Verification items for the finished model (mm, model axes). Face numbers are marked on the shaded views. Coordinates: 2 decimals unless noted, no trailing zeros. Write each loop counter-clockwise with the first axis right and the second up, starting at its lowest first coordinate (ties: lowest second). Pieces come first, ordered by that corner, then holes. Notation, with made-up numbers: (68.25, 71) -> (73.25, 71) arc R13 ccw to (73.25, 93) -> close; hole circle Ø10 at (71, -29). An arc over 180 degrees is marked (long way). Write item = value, one per line. Start each with the question number.
(1) Gauge pin test, flat ends, axial feed: pin 1 Ø3 at (y, z) = (-17, 3.5) entering from -X; pin 2 Ø2 at (y, z) = (33.5, 6) entering from -X. Record the tip position at first contact, or that the pin passes through.
(2) Mould release check, pull along X, two halves, no side actions. Record for the marked faces 1, 2 and 3: released by +X, released by -X, zero draft, split by the parting line, or undercut.
(3) Section check A-A (y = 0). State how many separate pieces and enclosed holes the cut face has, plus the area to 3 significant figures.
(4) Material ranges on probe 1 along Y at (x, z) = (25, 8); probe 2 along X at (y, z) = (7.5, 8); probe 3 along X at (y, z) = (-20, 6), recorded low to high. Write a range as [from, to].
(5) Section check B-B (z = 3.75). Record the cut outline in (x, y).
Autodesk Inventor part; units mm, degrees
ref_plane "YZ Plane" through (0, 0, 0) normal (1, 0, 0) x (0, 1, 0)
ref_plane "XZ Plane" through (0, 0, 0) normal (0, 1, 0) x (-1, 0, 0)
ref_plane "XY Plane" through (0, 0, 0) normal (0, 0, 1) x (1, 0, 0)
sketch "Sketch1" plane through (0, 0, 0) normal (0, 0, 1) x (1, 0, 0)
  circle A0 centre (0, 0) radius 46
  circle A1 centre (0, 0) radius 29.05
  dimension "d0" = 58.1
  dimension "d1" = 92
extrude "Extrusion1" add sketch "Sketch1" along normal blind 10
sketch "Sketch2" plane through (0, 0, 10) normal (0, 0, 1) x (1, 0, 0)
  circle A0 centre (0, 0) radius 29.05
  circle A1 centre (0, 0) radius 40 construction
  point P0 (0, 40)
  dimension "d4" = 80
hole "Hole1" at (0, 40, 10) direction (0, 0, -1) diameter 6.5 end through all
pattern_circular "Circular Pattern1" count 4 over 360 about axis through (0, 0, 0) along (0, 0, 1) of "Hole1"
sketch "Sketch4" plane through (0, 0, 10) normal (0, 0, 1) x (1, 0, 0)
  circle A0 centre (0, 0) radius 30
  circle A1 centre (0, 0) radius 34
  dimension "d15" = 60
  dimension "d16" = 68
extrude "Extrusion2" cut sketch "Sketch4" against normal blind 3
chamfer "Chamfer1" distance 0.4 angle 45 15 edges at (-46, 0, 0) (-46, 0, 10) (0, 43.25, 0) (-43.25, 0, 0) (43.25, 0, 0) (0, -43.25, 0) (43.25, 0, 10) (0, 43.25, 10) (0, -43.25, 10) (-43.25, 0, 10) (-29.05, 0, 0) (-34, 0, 10) (-34, 0, 7) (-30, 0, 7) (-30, 0, 10)
equation "\"d0\" = ID"
equation "\"d1\" = OD"
equation "\"OD\" = 92"
equation "\"ID\" = 58.1"
properties part number "pld_flange_groove_ak"
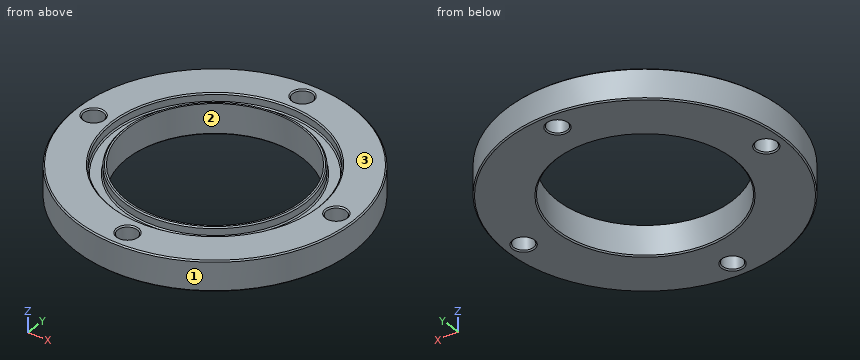
Response:
q1.pin_1 = -43.31
q1.pin_2 = -32.55
q2.face_1 = split by the parting line
q2.face_2 = undercut
q2.face_3 = zero draft
q3.separate_pieces = 4
q3.enclosed_holes = 0
q3.area = 184 mm2
q4.probe_1 = [-38.61, -23.04], [-16.58, -14.8], [14.8, 16.58], [23.04, 38.61]
q4.probe_2 = [-45.38, -33.16], [-29.05, -28.07], [28.07, 29.05], [33.16, 45.38]
q4.probe_3 = [-41.42, -21.07], [21.07, 41.42]
q5.outline = circle Ø92 at (0, 0); hole circle Ø6.5 at (-40, 0); hole circle Ø58.1 at (0, 0); hole circle Ø6.5 at (0, -40); hole circle Ø6.5 at (0, 40); hole circle Ø6.5 at (40, 0)
